Work out the finished part from the listing and answer in its coordinate system (mm). A direction names the side the tool comes from. Round coordinates to 2 decimals unless told otherwise and drop trailing zeros. Loops run counter-clockwise (first coordinate to the right, second up) from the corner with the lowest first, then second, coordinate; pieces in that order, holes last. Notation, with made-up numbers: M 69.5,39.5 L 94.5,39.5 A12 cw 94.5,52.5 Z; hole C 85.5,82.25 d7. An arc over 180 degrees is marked long. One line per item, written item: value.
Autodesk Inventor part; units mm, degrees
ref_plane "YZ Plane" through (0, 0, 0) normal (1, 0, 0) x (0, 1, 0)
ref_plane "XZ Plane" through (0, 0, 0) normal (0, 1, 0) x (-1, 0, 0)
ref_plane "XY Plane" through (0, 0, 0) normal (0, 0, 1) x (1, 0, 0)
sketch "Sketch1" plane through (0, 0, 0) normal (0, 0, 1) x (1, 0, 0)
  line L0 (5, -7.5) -> (-5, -7.5)
  line L1 (-5, -7.5) -> (-5, 7.5)
  line L2 (-5, 7.5) -> (5, 7.5)
  line L3 (5, 7.5) -> (5, -7.5)
  line L4 (5, -7.5) -> (-5, 7.5) construction
  line L5 (-5, -7.5) -> (5, 7.5) construction
  point P0 (0, 0)
  dimension "d0" = 10
  dimension "d1" = 15
extrude "Extrusion1" add sketch "Sketch1" against normal blind 1.6
sketch "Sketch2" plane through (0, 0, -1.6) normal (0, 0, -1) x (-1, 0, 0)
  circle A0 centre (0, 0) radius 3.45
  dimension "d4" = 6.9
extrude "Extrusion2" add sketch "Sketch2" along normal blind 1.4
fillet "Fillet1" radius 0.25 1 edges at (3.45, 0, -1.6)
fillet "Fillet2" radius 1.5 4 edges at (5, 7.5, -0.8) (-5, 7.5, -0.8) (-5, -7.5, -0.8) (5, -7.5, -0.8)
sketch "Sketch3" plane through (0, 0, -3) normal (0, 0, -1) x (-1, 0, 0)
  circle A0 centre (0, 0) radius 3.45
hole "Hole1" at (0, 0, -3) direction (0, 0, 1) diameter 4.134 end through all
fillet "Fillet3" radius 0.25 2 edges at (0, -2.067, 0) (0, -2.067, -3)
chamfer "Chamfer1" distance 0.1 angle 45 1 edges at (3.45, 0, -3)
chamfer "Chamfer2" distance 0.1 angle 45 16 edges at (4.5607, 7.0607, 0) (5, 0, 0) (4.5607, -7.0607, 0) (0, -7.5, 0) (-4.5607, -7.0607, 0) (-5, 0, 0) (-4.5607, 7.0607, 0) (0, 7.5, 0) (4.5607, 7.0607, -1.6) (0, 7.5, -1.6) (-4.5607, 7.0607, -1.6) (-5, 0, -1.6) (-4.5607, -7.0607, -1.6) (0, -7.5, -1.6) (4.5607, -7.0607, -1.6) (5, 0, -1.6)
properties part number "M5 T SLOT NUT"
1) Find section D-D (y = 4). Give the vertices of the cut face in (x, z), then the cut area to 3 significant figures.
Check values:
outline: M -5,-1.5 L -4.9,-1.6 L 4.9,-1.6 L 5,-1.5 L 5,-0.1 L 4.9,0 L -4.9,0 L -5,-0.1 Z
area: 16.0 mm2
2) Find section C-C (z = -0.8). Give the vertices of the cut face in (x, y), then the cut area to 3 significant figures.
Check values:
outline: M -5,-6 A1.5 ccw -3.5,-7.5 L 3.5,-7.5 A1.5 ccw 5,-6 L 5,6 A1.5 ccw 3.5,7.5 L -3.5,7.5 A1.5 ccw -5,6 Z; hole C 0,0 d4.13
area: 135 mm2
3) Find section A-A (y = 0). Give the vertices of the cut face in (x, z), then the cut area to 3 significant figures.
Check values:
outline: M -5,-1.5 L -4.9,-1.6 L -3.7,-1.6 A0.25 cw -3.45,-1.85 L -3.45,-2.9 L -3.35,-3 L -2.32,-3 A0.25 ccw -2.07,-2.75 L -2.07,-0.25 A0.25 ccw -2.32,0 L -4.9,0 L -5,-0.1 Z; M 2.07,-2.75 A0.25 ccw 2.32,-3 L 3.35,-3 L 3.45,-2.9 L 3.45,-1.85 A0.25 cw 3.7,-1.6 L 4.9,-1.6 L 5,-1.5 L 5,-0.1 L 4.9,0 L 2.32,0 A0.25 ccw 2.07,-0.25 Z
area: 13.2 mm2
4) Find the intervals of material crossed by probe 1 along Y at (x, z) = (0, -1.85); probe 2 along Y at (x, z) = (0, -0.75); probe 3 along Z at (x, y) = (2.25, 6.5), in increasing order. Write a range as from..to.
Check values:
probe 1: -3.45..-2.07, 2.07..3.45
probe 2: -7.5..-2.07, 2.07..7.5
probe 3: -1.6..0
5) For faces 1 (the face through (-4.57, 7.05, -0.81)), 2 (the face through (-2.2, 3.4, -1.6)), determine the directions among +Z, -Z, +X, -X, +Y, -Y from which every point of the face is accessible in a straight line to the end or side of a thin tool.
Check values:
face 1: +Z, -Z, -X, +Y
face 2: -Z
6) Find section B-B (x = 0). Give the vertices of the cut face in (y, z), then the cut area to 3 significant figures.
Check values:
outline: M -7.5,-1.5 L -7.4,-1.6 L -3.7,-1.6 A0.25 cw -3.45,-1.85 L -3.45,-2.9 L -3.35,-3 L -2.32,-3 A0.25 ccw -2.07,-2.75 L -2.07,-0.25 A0.25 ccw -2.32,0 L -7.4,0 L -7.5,-0.1 Z; M 2.07,-2.75 A0.25 ccw 2.32,-3 L 3.35,-3 L 3.45,-2.9 L 3.45,-1.85 A0.25 cw 3.7,-1.6 L 7.4,-1.6 L 7.5,-1.5 L 7.5,-0.1 L 7.4,0 L 2.32,0 A0.25 ccw 2.07,-0.25 Z
area: 21.2 mm2
